from build123d import *

# Parameters (mm, degrees)
SKETCH2_W            = 14
SKETCH2_H            = 14
SKETCH2_W_2          = 4
SKETCH2_H_2          = 56
SKETCH2_W_3          = 5
SKETCH2_H_3          = 43
SKETCH2_H_4          = 5
KEY_PLATE_DEPTH      = 1.5
SKETCH4_W            = 10
SKETCH4_H            = 10
SKETCH4_W_2          = 7
SKETCH4_H_2          = 7
SKETCH4_H_3          = 4.796695527
SKETCH4_H_4          = 4.186773245
SKETCH4_W_3          = 15
SKETCH4_W_4          = 20.633111118
SKETCH4_H_5          = 5
STANDOFFS_DEPTH      = 3.5
SKETCH6_R            = 5
SCREW_GUIDES_DEPTH   = 3.5
M3_CLEARANCE_HOLE1_D = 3.2


with BuildPart() as part:
    # Sketch2 → Key Plate (new body)
    with BuildSketch(Plane(origin=(0, 0, 0), x_dir=(1, 0, 0), z_dir=(0, 1, 0))):
        Polygon((-132.282827099, 11.085546756), (-132.282827099, 68.085546756), (-100.898050788, 81.085546756), (-55.483837226, 81.085546756), (-41.483837226, 67.085546756), (-8.649715981, 67.085546756), (-8.649715981, 77.800355514), (7.371180312, 84.43642804), (73.386249254, 67.093850916), (73.386249254, 39.093850916), (59.91832331, 39.093850916), (-2.282827099, 13.329290821), (-2.282827099, -27.914453244), (-36.282827099, -27.914453244), (-66.282827099, -11.897922016), (-66.282827099, 11.085546756), align=None)
        Polygon((5.863113655, 38.297174055), (-7.0711998, 32.939606002), (-12.428767853, 45.873919457), (0.505545602, 51.23148751), align=None, mode=Mode.SUBTRACT)
        with Locations((-118.282827099, 54.085546756)):
            Rectangle(SKETCH2_W, SKETCH2_H, mode=Mode.SUBTRACT)
        with Locations((-90.282827099, 67.085546756)):
            Rectangle(SKETCH2_W, SKETCH2_H, mode=Mode.SUBTRACT)
        with Locations((-61.282827099, 67.085546756)):
            Rectangle(SKETCH2_W, SKETCH2_H, mode=Mode.SUBTRACT)
        with Locations((-36.282827099, 53.085546756)):
            Rectangle(SKETCH2_W, SKETCH2_H, mode=Mode.SUBTRACT)
        with Locations((-61.282827099, 38.085546756)):
            Rectangle(SKETCH2_W, SKETCH2_H, mode=Mode.SUBTRACT)
        with Locations((-90.282827099, 38.085546756)):
            Rectangle(SKETCH2_W, SKETCH2_H, mode=Mode.SUBTRACT)
        with Locations((-118.282827099, 25.085546756)):
            Rectangle(SKETCH2_W, SKETCH2_H, mode=Mode.SUBTRACT)
        with Locations((-52.282827099, -0.101226489)):
            Rectangle(SKETCH2_W, SKETCH2_H, mode=Mode.SUBTRACT)
        with Locations((-36.282827099, 24.085546756)):
            Rectangle(SKETCH2_W, SKETCH2_H, mode=Mode.SUBTRACT)
        with Locations((-19.282827099, -10.914453244)):
            Rectangle(SKETCH2_W, SKETCH2_H, mode=Mode.SUBTRACT)
        with Locations((59.386249254, 53.093850916)):
            Rectangle(SKETCH2_W, SKETCH2_H, mode=Mode.SUBTRACT)
        Polygon((-3.649715981, 74.459462324), (9.284597474, 79.817030378), (14.642165527, 66.882716922), (1.707852072, 61.525148869), align=None, mode=Mode.SUBTRACT)
        Polygon((3.640403405, 56.85955723), (16.57471686, 62.217125283), (21.932284914, 49.282811828), (8.997971458, 43.925243775), align=None, mode=Mode.SUBTRACT)
        Polygon((26.597876553, 51.215363162), (39.532190008, 56.572931215), (34.174621955, 69.50724467), (21.2403085, 64.149676617), align=None, mode=Mode.SUBTRACT)
        Polygon((-24.282827099, 62.085546756), (-3.936233335, 62.085546756), (-1.361677583, 55.870019344), (-24.282827099, 46.37576835), align=None, mode=Mode.SUBTRACT)
        with Locations((-104.282827099, 46.085546756)):
            Rectangle(SKETCH2_W_2, SKETCH2_H_2, mode=Mode.SUBTRACT)
        with Locations((-75.782827099, 52.585546756)):
            Rectangle(SKETCH2_W_3, SKETCH2_H_3, mode=Mode.SUBTRACT)
        with Locations((-90.282827099, 52.585546756)):
            Rectangle(SKETCH2_W, SKETCH2_H_4, mode=Mode.SUBTRACT)
        with Locations((-61.282827099, 52.585546756)):
            Rectangle(SKETCH2_W, SKETCH2_H_4, mode=Mode.SUBTRACT)
        with Locations((-36.282827099, 38.585546756)):
            Rectangle(SKETCH2_W, SKETCH2_H_4, mode=Mode.SUBTRACT)
        with Locations((-118.282827099, 39.585546756)):
            Rectangle(SKETCH2_W, SKETCH2_H_4, mode=Mode.SUBTRACT)
        Polygon((19.280697361, 68.749940108), (30.195022846, 73.270801748), (15.846767853, 77.040179298), align=None, mode=Mode.SUBTRACT)
    extrude(amount=KEY_PLATE_DEPTH)

    # Sketch4 → Standoffs (add)
    with BuildSketch(Plane.XZ.offset(-1.5)):
        with Locations((-7.282827099, 22.914453244)):
            Rectangle(SKETCH4_W, SKETCH4_H)
        with Locations((69.886249254, -42.593850916)):
            Rectangle(SKETCH4_W_2, SKETCH4_H_2)
        with Locations((69.886249254, -63.593850916)):
            Rectangle(SKETCH4_W_2, SKETCH4_H_2)
        with Locations((-128.782827099, -14.585546756)):
            Rectangle(SKETCH4_W_2, SKETCH4_H_2)
        with Locations((-128.782827099, -64.585546756)):
            Rectangle(SKETCH4_W_2, SKETCH4_H_2)
        with Locations((-62.782827099, 9.499574253)):
            Rectangle(SKETCH4_W_2, SKETCH4_H_3)
        with Locations((-31.282827099, 22.914453244)):
            Rectangle(SKETCH4_W, SKETCH4_H)
        with Locations((-62.782827099, -8.992160134)):
            Rectangle(SKETCH4_W_2, SKETCH4_H_4)
        with Locations((-75.782827099, -77.585546756)):
            Rectangle(SKETCH4_W_3, SKETCH4_H_2)
        with Locations((-18.96627154, -64.585546756)):
            Rectangle(SKETCH4_W_4, SKETCH4_H_5)
    extrude(amount=-STANDOFFS_DEPTH)

    # Sketch6 → Screw Guides (add)
    with BuildSketch(Plane.XZ.offset(-1.5)):
        with Locations((22.140830524, -30.487456679)):
            Circle(SKETCH6_R)
        with Locations((-13.803783609, -15.564500098)):
            Circle(SKETCH6_R)
        with Locations((-75.782827099, -20.294986151)):
            Circle(SKETCH6_R)
    extrude(amount=-SCREW_GUIDES_DEPTH)

    # M3 Clearance Hole1 (through all)
    with Locations(Plane(origin=(22.140830524, 5, -30.487456679), x_dir=(0, 0, 1), z_dir=(0, 1, 0))):
        with Locations((0, 0), (10.192470528, -97.923657623), (14.922956581, -35.944614133)):
            Hole(M3_CLEARANCE_HOLE1_D / 2)


solid = part.part
Geometry: final body of the model. Coordinates: model frame, mm. A direction names the side the tool comes from. Round coordinates to 2 decimals unless told otherwise and drop trailing zeros. Loops run counter-clockwise (first coordinate to the right, second up) from the corner with the lowest first, then second, coordinate; pieces in that order, holes last. Notation, with made-up numbers: (9.25, -1.5) -> (33.25, -1.5) arc R18 cw to (33.25, 21.5) -> close; hole circle Ø8 at (-12, 58). An arc over 180 degrees is marked (long way). One line per question, with ' | ' between items. Start each with the question number.
1. Contact query for flat-ended pins moving along their axis: pin 1 (1 mm diameter, centred on x = -73.5, z = -42.5, fed in from +Y); pin 2 (1.8 mm diameter, centred on x = -62, y = 3, fed in from +Z); pin 3 (1.6 mm diameter, centred on y = 0.5, z = -23, fed in from +X). Output: stop coordinate, or through.
2. Mould query, pull axis X, two halves, no side actions, for faces 6 (the face through (-19, 1.5, 23)), 7 (the face through (70, 1.5, -53)), 8 (the face through (29.25, 0.74, -26.39)). Classes: pulls with the +X half, pulls with the -X half, needs draft (parallel to the pull), parting line crosses it, or undercut.
3. Set-up query: faces 1 (the face through (-79, 2, -81.086)), 2 (the face through (-9.712, 0.74, -39.316)), 3 (the face through (-76, 3, -74.086)), 4 (the face through (-129, 5, -65)), 5 (the face through (-20, 1, 27.914)). Return all of +Z, -Z, +X, -X, +Y, -Y with unobstructed straight access to the full face (end or side cutting, diameter ignored); none if empty.
4. Section A-A on x = -33.5. Output: boundary loops of the cut face in (y, z).
5. Section C-C on x = 48.5. Output: boundary loops of the cut face in (y, z).
6. Line query: line 1 along X through (y, z) = (0.6, -25.5); line 2 along Z through (x, y) = (-36, 0.8); line 3 along Z through (x, y) = (-65, 3.7). Output: solid intervals per line, ascending. Write a range as [from, to].
7. Section B-B on y = 2.9. Count the separate pieces of the cut face and the enclosed holes in it, and give its area (3 significant figures).
Returned:
1) pin 1: stops at y = 1.5 | pin 2: stops at z = 11.9 | pin 3: stops at x = 23
2) face 6: undercut | face 7: needs draft | face 8: pulls with the +X half
3) face 1: -Z, -X, +Y, -Y | face 2: +Y, -Y | face 3: +Y | face 4: +Z, -Z, +X, -X, +Y | face 5: +Z, +X, -X, +Y, -Y
4) outline: (0, -67.09) -> (1.5, -67.09) -> (1.5, -60.09) -> (0, -60.09) -> close; (0, -46.09) -> (1.5, -46.09) -> (1.5, -41.09) -> (0, -41.09) -> close; (0, -36.09) -> (1.5, -36.09) -> (1.5, -31.09) -> (0, -31.09) -> close; (0, -17.09) -> (1.5, -17.09) -> (1.5, 17.91) -> (5, 17.91) -> (5, 27.91) -> (0, 27.91) -> close
5) outline: (0, -73.63) -> (1.5, -73.63) -> (1.5, -34.36) -> (0, -34.36) -> close
6) line 1: x = [-132.28, -125.28], [-111.28, -106.28], [-102.28, -43.28], [-29.28, 27.1] | line 2: z = [-67.09, -60.09], [-46.09, -41.09], [-36.09, -31.09], [-17.09, 27.91] | line 3: z = [-11.09, -6.9], [7.1, 11.9]
7) separate pieces: 13 | enclosed holes: 3 | area: 879 mm2
